Check sheet for the modelled part. Datum: model origin and axes. Units: mm. Face numbers are marked on the shaded views. Give positions to 0.01 mm unless a question says otherwise; leave off trailing zeros. Order: outer loops, then holes, each group sorted by start corner. A loop starts at its lowest first (then second) coordinate and runs counter-clockwise, first axis right, second up.
from build123d import *

# Parameters (mm, degrees)
SKETCH1_R           = 27.5
BOSS_EXTRUDE1_DEPTH = 5.08
SKETCH2_R           = 1.025
CUT_EXTRUDE1_DEPTH  = 3.175
SKETCH3_R           = 3.095
CUT_EXTRUDE2_DEPTH  = 40.221249343


with BuildPart() as part:
    # Sketch1 → Boss-Extrude1 (new body)
    with BuildSketch(Plane(origin=(0, 0, 0), x_dir=(1, 0, 0), z_dir=(0, 1, 0))):
        with Locations(Location((0, 0, 0), (0, 0, 270))):
            Circle(SKETCH1_R)
    extrude(amount=BOSS_EXTRUDE1_DEPTH)

    # Sketch2 → Cut-Extrude1 (cut)
    with BuildSketch(Plane(origin=(0, 5.08, 0), x_dir=(1, 0, 0), z_dir=(0, 1, 0))):
        with Locations(Location((16.164461018, 16.164461018, 0), (0, 0, 270))):
            Circle(SKETCH2_R)
        with Locations(Location((16.164461018, -16.164461018, 0), (0, 0, 270))):
            Circle(SKETCH2_R)
        with Locations(Location((-16.164461018, -16.164461018, 0), (0, 0, 270))):
            Circle(SKETCH2_R)
        with Locations(Location((-16.164461018, 16.164461018, 0), (0, 0, 270))):
            Circle(SKETCH2_R)
    extrude(amount=-CUT_EXTRUDE1_DEPTH, mode=Mode.SUBTRACT)

    # Sketch3 → Cut-Extrude2 (cut, through all)
    with BuildSketch(Plane(origin=(0, 5.08, 0), x_dir=(1, 0, 0), z_dir=(0, 1, 0))):
        with Locations(Location((-6.35, 0, 0), (0, 0, 270))):
            Circle(SKETCH3_R)
        with Locations(Location((16.51, 0, 0), (0, 0, 270))):
            Circle(SKETCH3_R)
    extrude(amount=-CUT_EXTRUDE2_DEPTH, mode=Mode.SUBTRACT)


solid = part.part
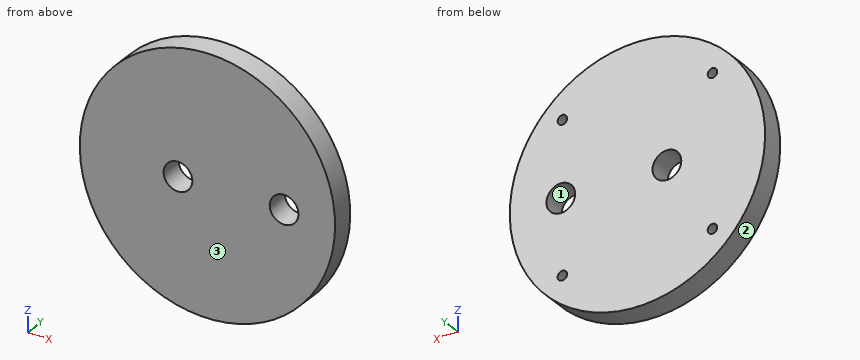
1) Depth check by flat-ended pin: pin 1 Ø1 at (x, z) = (16.5, -16.5) entering from +Y (3 decimals); pin 2 Ø1.6 at (x, z) = (-16.5, -15.5) entering from +Y. Enter the tip coordinate at first touch or a pass-through.
Recorded:
pin 1: stops at y = 1.905
pin 2: stops at y = 5.08
2) Section check D-D, the plane y = 0.9. Record the cut outline in (x, z) (3 decimals).
Recorded:
outline: circle Ø55 at (0, 0); hole circle Ø6.19 at (-6.35, 0); hole circle Ø6.19 at (16.51, 0)
3) Section check A-A, the plane z = 0. Record the cut outline in (x, y) (3 decimals).
Recorded:
outline: (-27.5, 0) - (-9.445, 0) - (-9.445, 5.08) - (-27.5, 5.08) - close; (-3.255, 0) - (13.415, 0) - (13.415, 5.08) - (-3.255, 5.08) - close; (19.605, 0) - (27.5, 0) - (27.5, 5.08) - (19.605, 5.08) - close
4) Material ranges on L1, parallel to X at y = 3, z = 0 (3 decimals); L2, parallel to X at y = 4.1, z = -17; L3, parallel to Z at x = 19, y = 0.9, recorded low to high.
Recorded:
L1: x = -27.5 to -9.445, -3.255 to 13.415, 19.605 to 27.5
L2: x = -21.62 to -16.76, -15.57 to 15.57, 16.76 to 21.62
L3: z = -19.88 to -1.84, 1.84 to 19.88
5) Section check C-C, the plane x = -6.35. Record the cut outline in (y, z) (3 decimals).
Recorded:
outline: (0, -26.757) - (5.08, -26.757) - (5.08, -3.095) - (0, -3.095) - close; (0, 3.095) - (5.08, 3.095) - (5.08, 26.757) - (0, 26.757) - close
6) Section check B-B, the plane y = 4.1. Record the cut outline in (x, z) (3 decimals).
Recorded:
outline: circle Ø55 at (0, 0); hole circle Ø2.05 at (-16.164, -16.164); hole circle Ø2.05 at (-16.164, 16.164); hole circle Ø6.19 at (-6.35, 0); hole circle Ø6.19 at (16.51, 0); hole circle Ø2.05 at (16.164, -16.164); hole circle Ø2.05 at (16.164, 16.164)
7) Draft check along X on the marked faces 1, 2 and 3. Enter one of: +X half, -X half, draft (parallel to the pull), parting line (faces both ways), or undercut.
Recorded:
face 1: undercut
face 2: parting line
face 3: draft
